CAD build for the part. Positions are in the model's coordinates, mm. A direction names the side the tool comes from. Coordinates: 2 decimals unless noted, no trailing zeros. Order: outer loops, then holes, each group sorted by start corner. A loop starts at its lowest first (then second) coordinate and runs counter-clockwise, first axis right, second up. Notation, with made-up numbers: (0, 6.5) - (19, 6.5) arc R35 cw to (19, 44.5) - close; hole circle Ø1 at (-8.75, -3). An arc over 180 degrees is marked (long way). Return JSON: item names as keys, results as strings.
from build123d import *

# Parameters (mm, degrees)
F0_W      = 30.1244
F0_H      = 20.5486
F1_DEPTH  = 4.064
F2_W      = 11.7348
F2_H      = 13.4112
F3_DEPTH  = 10.16
F4_R      = 4.1148
F5_DEPTH  = 7.62
F6_W      = 1.714757
F6_H      = 6.894373
F6_H_2    = 6.894372
F5_FACE_R = 4.1148
F7_DEPTH  = 1.27


with BuildPart() as f1:
    # F0 (on Top) → F1 (new body)
    with BuildSketch(Plane.XY):
        Rectangle(F0_W, F0_H)
    extrude(amount=F1_DEPTH)

    # F2 (on face) → F3 (join)
    with BuildSketch(Plane.XY.offset(4.064)):
        Rectangle(F2_W, F2_H)
    extrude(amount=F3_DEPTH)



with BuildPart() as f5:
    # F4 (on Front) → F5 (new body, symmetric)
    with BuildSketch(Plane.XZ):
        with Locations((10.4902, 9.144)):
            Circle(F4_R)
        with Locations((-10.4902, 9.144)):
            Circle(F4_R)
    extrude(amount=F5_DEPTH, both=True)


with BuildPart() as f1_1:
    add(f1.part)

    add(f5.part)  # F7 merges F5
    # F6 (on Front) + F5_face (on face) → F7 (join, symmetric)
    with BuildSketch(Plane.XZ):
        with Locations((-10.485539, 5.029202)):
            Rectangle(F6_W, F6_H)
        with Locations((10.657787, 5.032614)):
            Rectangle(F6_W, F6_H_2)
    with BuildSketch(Plane(origin=(10.4902, -7.62, 9.144), x_dir=(1, 0, 0), z_dir=(0, -1, 0))):
        Circle(F5_FACE_R)
    extrude(amount=F7_DEPTH, both=True)


solid = f1_1.part
Item 1: Mould opens along Z. For faces 4 (the flat face through (-11.343, 0, 4.6)), 5 (the flat face through (10, -8.89, 9)), 6 (the flat face through (11.515, 0, 5)), 7 (the flat face through (0, 0, 14.224)) say: released by +Z, released by -Z, zero draft, split by the parting line, or undercut.
Findings below:
{"face 4": "undercut", "face 5": "zero draft", "face 6": "undercut", "face 7": "released by +Z"}
Item 2: Wall check: L1, parallel to X at y = 4.25, z = 9.25; L2, parallel to X at y = -1, z = 4.5; L3, parallel to Z at x = -0.5, y = 7. Give the ranges that are in metal, low to high. Write a range as [from, to].
Findings below:
{"L1": "x = [-14.6, -6.38], [-5.87, 5.87], [6.38, 14.6]", "L2": "x = [-11.34, -9.63], [-5.87, 5.87], [9.8, 11.52]", "L3": "z = [0, 4.06]"}
Item 3: Band-saw the part on A-A, the plane x = -5. List the corners of the cut face in (y, z).
Findings below:
{"outline": "(-10.27, 0) - (10.27, 0) - (10.27, 4.06) - (6.71, 4.06) - (6.71, 14.22) - (-6.71, 14.22) - (-6.71, 4.06) - (-10.27, 4.06) - close"}
Item 4: Band-saw the part on C-C, the plane y = -5. List the corners of the cut face in (x, z) (3 decimals).
Findings below:
{"outline": "(-15.062, 0) - (15.062, 0) - (15.062, 4.064) - (5.867, 4.064) - (5.867, 14.224) - (-5.867, 14.224) - (-5.867, 4.064) - (-15.062, 4.064) - close; circle Ø8.23 at (-10.49, 9.144); circle Ø8.23 at (10.49, 9.144)"}
Item 5: Which spindle directions (+Z, -Z, +X, -X, +Y, -Y) get a long thin tool onto all of the face, cutting with end or side? Do faces 1 (the flat face through (-11, -7.62, 9)), 2 (the flat face through (9.8, 0, 4.6)), 3 (the flat face through (-5.867, 0, 9)). Say none if no direction does.
Findings below:
{"face 1": "+Z, -X, -Y", "face 2": "+Y, -Y", "face 3": "+Z, +Y, -Y"}
Item 6: Band-saw the part on D-D, the plane z = 7.25. List the corners of the cut face in (x, y), then the cut area to 3 significant figures.
Findings below:
{"outline": "(-14.14, -7.62) - (-6.84, -7.62) - (-6.84, 7.62) - (-14.14, 7.62) - close; (-5.87, -6.71) - (5.87, -6.71) - (5.87, 6.71) - (-5.87, 6.71) - close; (6.84, -8.89) - (14.14, -8.89) - (14.14, 7.62) - (6.84, 7.62) - close", "area": "389 mm²"}
Item 7: Band-saw the part on B-B, the plane z = 10.5. List the corners of the cut face in (x, y), then the cut area to 3 significant figures.
Findings below:
{"outline": "(-14.38, -7.62) - (-6.61, -7.62) - (-6.61, 7.62) - (-14.38, 7.62) - close; (-5.87, -6.71) - (5.87, -6.71) - (5.87, 6.71) - (-5.87, 6.71) - close; (6.61, -8.89) - (14.38, -8.89) - (14.38, 7.62) - (6.61, 7.62) - close", "area": "404 mm²"}
Item 8: Drop flat-ended pins along their axis: P1, Ø5, axis at y = 1.5, z = 11, coming from the -X side (3 decimals); P2, Ø8, axis at x = 11, y = 1, coming from the +Z side; P3, Ø1.5, axis at x = 9, y = -5, coming from the +Z side. Give the stop position or say it passes through.
Findings below:
{"P1": "stops at x = -14.605", "P2": "stops at z = 13.26", "P3": "stops at z = 13.19"}
